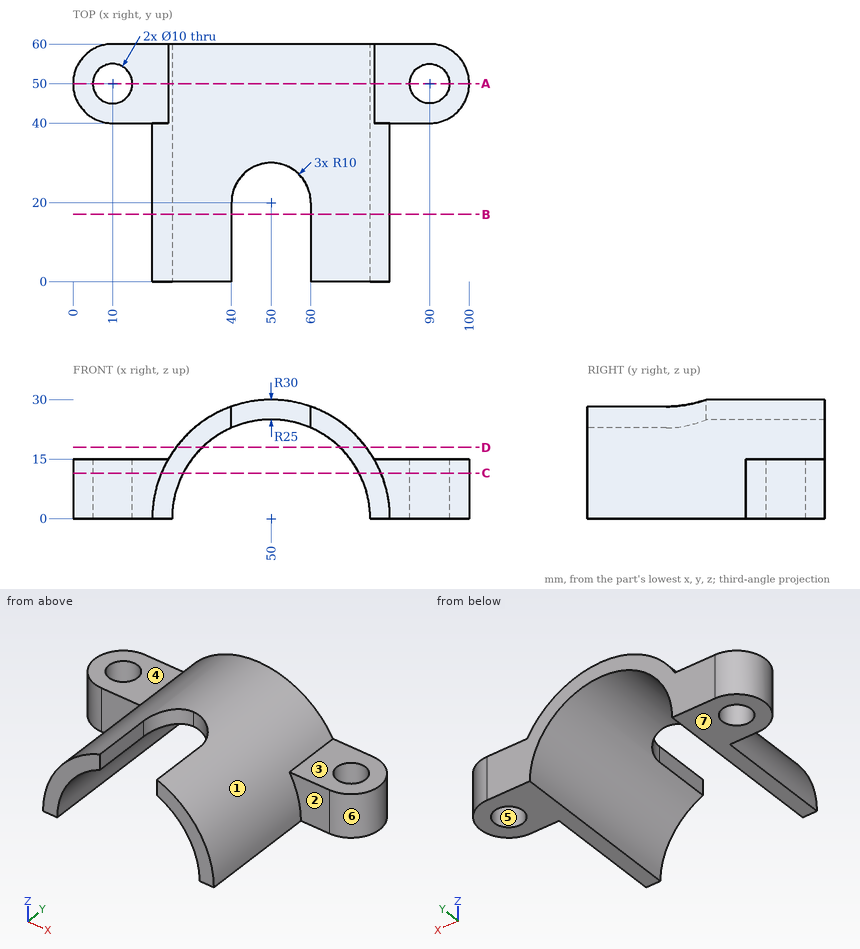
Geometry: see drawing. Coordinates: mm, zero at the bounding-box minimum. A direction names the side the tool comes from. Round coordinates to 2 decimals unless told otherwise and drop trailing zeros. Write each loop counter-clockwise with the first axis right and the second up, starting at its lowest first coordinate (ties: lowest second). Pieces come first, ordered by that corner, then holes.
Item 1: Mould query, pull axis X, two halves, no side actions, for the marked faces 5, 6 and 7. Classes: +X half, -X half, draft (parallel to the pull), parting line (faces both ways), or undercut.
Item 2: Section query B-B (y = 17). Return loops of the section in (x, z).
Item 3: Set-up query: the marked faces 1, 2, 3 and 4. Return all of +Z, -Z, +X, -X, +Y, -Y with unobstructed straight access to the full face (end or side cutting, diameter ignored); none if empty.
Item 4: Section query A-A (y = 50). Return loops of the section in (x, z), plus the area to 3 significant figures.
Item 5: Material intervals for L1, parallel to Y at x = 10, z = 3; L2, parallel to X at y = 47, z = 23; L3, parallel to X at y = 9.5, z = 6, sorted ascending.
Item 6: Section query C-C (z = 11.5). Return loops of the section in (x, y).
Item 7: Pin query (flat end, axial travel): P1, Ø4, axis at y = 18, z = 18.5, coming from the -X side; P2, Ø7, axis at x = 15, z = 4.5, coming from the -Y side; P3, Ø3, axis at x = 35, y = 18, coming from the +Z side. Return the tip coordinate at first contact, or that it passes through.
Item 8: Section query D-D (z = 18). Return loops of the section in (x, y), plus the area to 3 significant figures.
Completed:
1. face 5: undercut
1. face 6: +X half
1. face 7: draft
2. outline: (20, 0) - (25, 0) arc R25 cw to (40, 22.91) - (40, 28.28) arc R30 ccw to start; (60, 22.91) arc R25 cw to (75, 0) - (80, 0) arc R30 ccw to (60, 28.28) - close
3. face 1: +Z, -Y
3. face 2: +Z, +X, -Y
3. face 3: +Z, +X, +Y, -Y
3. face 4: +Z, -X, +Y, -Y
4. outline: (0, 0) - (5, 0) - (5, 15) - (0, 15) - close; (15, 0) - (25, 0) arc R25 cw to (75, 0) - (85, 0) - (85, 15) - (75.98, 15) arc R30 ccw to (24.02, 15) - (15, 15) - close; (95, 0) - (100, 0) - (100, 15) - (95, 15) - close
4. area: 771 mm2
5. L1: y = 40 to 45, 55 to 60
5. L2: x = 30.74 to 40.2, 59.8 to 69.26
5. L3: x = 20.61 to 25.73, 74.27 to 79.39
6. outline: (10, 40) - (22.29, 40) - (22.29, 0) - (27.8, 0) - (27.8, 60) - (10, 60) arc R10 ccw to start; (72.2, 0) - (77.71, 0) - (77.71, 40) - (90, 40) arc R10 ccw to (90, 60) - (72.2, 60) - close; hole circle Ø10 at (10, 50); hole circle Ø10 at (90, 50)
7. P1: stops at x = 24.95
7. P2: stops at y = 40
7. P3: stops at z = 26.79
8. outline: (26, 0) - (32.65, 0) - (32.65, 60) - (26, 60) - close; (67.35, 0) - (74, 0) - (74, 60) - (67.35, 60) - close
8. area: 798 mm2
